from build123d import *

# Parameters (mm, degrees)
F0_W     = 600
F0_H     = 800
F1_DEPTH = 600
F2_T     = -17
F4_W     = 566
F4_H     = 483
F5_DEPTH = 17


with BuildPart() as f1:
    # F0 (on Front) → F1 (new body)
    with BuildSketch(Plane.XZ):
        with Locations((300, 400)):
            Rectangle(F0_W, F0_H)
    extrude(amount=F1_DEPTH)

    # F2
    f2_openings = [f1.faces().sort_by_distance(p)[0] for p in [
        (300, -600, 400),
    ]]
    offset(amount=F2_T, openings=f2_openings)

    # F4 (on face) → F5 (cut, through all)
    with BuildSketch(Plane.XY.offset(800)):
        with Locations((300, -258.5)):
            Rectangle(F4_W, F4_H)
    extrude(amount=-F5_DEPTH, mode=Mode.SUBTRACT)


solid = f1.part
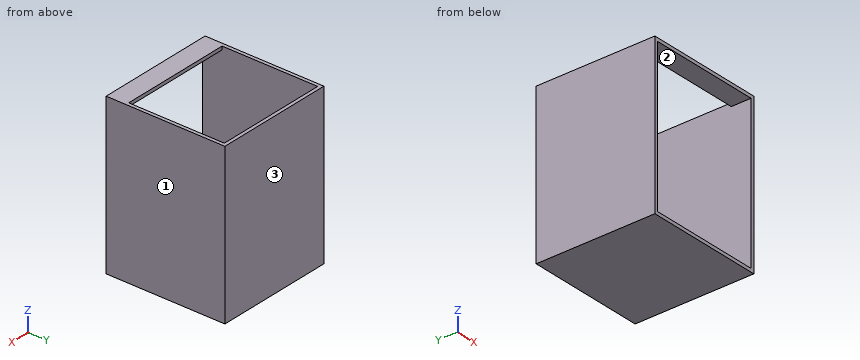
Read the model definition and answer for the solid it produces. Units are mm, in the model's axes. Face numbers are marked on the shaded views. Round coordinates to 2 decimals unless told otherwise and drop trailing zeros. Write each loop counter-clockwise with the first axis right and the second up, starting at its lowest first coordinate (ties: lowest second). Pieces come first, ordered by that corner, then holes.
1. Given pin 1 Ø12 at (x, z) = (112, 334.5) entering from -Y, flat-ended and moving along its own axis, determine where the tip first touches the part or whether it passes through.
2. The part is cut by section C-C, the plane z = 137.5. Determine the outline of the cut face in (x, y), then the cut area to 3 significant figures.
3. Straight lines are drawn through the part: L1, parallel to X at y = -559.5, z = 178; L2, parallel to Z at x = 532, y = -274; L3, parallel to Y at x = 512, z = 479. For each, find the intervals that lie inside material, in ascending order.
4. The part is cut by section B-B, the plane y = -96.5. Determine the outline of the cut face in (x, z), then the cut area to 3 significant figures.
5. Determine the mould class of the marked faces 1, 2 and 3 for opening direction X: pulls with the +X half, pulls with the -X half, needs draft (parallel to the pull), parting line crosses it, or undercut.
6. The part is cut by section A-A, the plane x = 497. Determine the outline of the cut face in (y, z), then the cut area to 3 significant figures.
Values:
1. pin 1: stops at y = -17
2. outline: (0, -600) - (17, -600) - (17, -17) - (583, -17) - (583, -600) - (600, -600) - (600, 0) - (0, 0) - close
2. area: 30,000 mm2
3. L1: x = 0 to 17, 583 to 600
3. L2: z = 0 to 17
3. L3: y = -17 to 0
4. outline: (0, 0) - (600, 0) - (600, 800) - (583, 800) - (583, 17) - (17, 17) - (17, 800) - (0, 800) - close
4. area: 36,800 mm2
5. face 1: pulls with the +X half
5. face 2: undercut
5. face 3: needs draft
6. outline: (-600, 0) - (0, 0) - (0, 800) - (-17, 800) - (-17, 17) - (-600, 17) - close; (-600, 783) - (-500, 783) - (-500, 800) - (-600, 800) - close
6. area: 25,200 mm2
